Geometry: final body of the model. Coordinates: model frame, mm. A direction names the side the tool comes from. Give positions to 0.01 mm unless a question says otherwise; leave off trailing zeros. Write each loop counter-clockwise with the first axis right and the second up, starting at its lowest first coordinate (ties: lowest second). Pieces come first, ordered by that corner, then holes. Notation, with made-up numbers: (68, 47) -> (102, 47) arc R33 cw to (102, 83) -> close; hole circle Ø8 at (34.5, 2). An arc over 180 degrees is marked (long way). Use CSV: the item, a comma, the result in double quotes. Start each with the question number.
1) Set-up query: faces 1 (the face through (14, 5, 2)), 2 (the face through (2, 27.42, 2)), 3 (the face through (26, 19.42, 2)), 4 (the face through (19.5, 35, 2)), 5 (the face through (8, 35, 2)). Return all of +Z, -Z, +X, -X, +Y, -Y with unobstructed straight access to the full face (end or side cutting, diameter ignored); none if empty.
2) Section C-C (z = 3). Output: boundary loops of the cut face in (x, y), plus the area to 3 significant figures.
3) Section A-A (y = 19). Output: boundary loops of the cut face in (x, z).
4) Material intervals for line 1 (Y direction, x = 13.75, z = 2.6); line 2 (Y direction, x = 24.49, z = 1.7); line 3 (X direction, y = 14.5, z = 3.65), sorted ascending. Write a range as [from, to].
5) Section D-D (x = 4.5). Output: boundary loops of the cut face in (y, z), plus the area to 3 significant figures.
6) Contact query for flat-ended pins moving along their axis: P1, Ø2, axis at x = 2.5, z = 2.5, coming from the -Y side; P2, Ø1, axis at x = 24.5, z = 1, coming from the +Y side; P3, Ø2, axis at y = 35, z = 1.5, coming from the -X side. Output: stop coordinate, or through.
7) Section B-B (x = 24). Output: boundary loops of the cut face in (y, z), plus the area to 3 significant figures.
8) Draft query along Y for faces 6 (the face through (4, 32.42, 2)), 7 (the face through (2, 2.1, 2)), 8 (the face through (2, 19.42, 2)), 9 (the face through (25, 27.42, 2)). Return one class per face: pulls with the +Y half, pulls with the -Y half, needs draft (parallel to the pull), parting line crosses it, or undercut.
```python
from build123d import *

# Parameters (mm, degrees)
SKETCH1_R           = 1.2
SKETCH1_W           = 12.42
SKETCH1_H           = 22.42
BOSS_EXTRUDE1_DEPTH = 4
FILLET1_R           = 7


with BuildPart() as part:
    # Sketch1 → Boss-Extrude1 (new body)
    with BuildSketch(Plane.XY):
        Polygon((8, 37.42), (8, 32.42), (0, 32.42), (0, 27.42), (4, 27.42), (4, 19.42), (0, 19.42), (0, 0), (27.5, 0), (27.5, 19.42), (23.5, 19.42), (23.5, 27.42), (27.5, 27.42), (27.5, 32.42), (19.5, 32.42), (19.5, 37.42), align=None)
        with Locations((4, 13)):
            Circle(SKETCH1_R, mode=Mode.SUBTRACT)
        with Locations((13.75, 16.21)):
            Rectangle(SKETCH1_W, SKETCH1_H, mode=Mode.SUBTRACT)
        with Locations((24.49, 13.01)):
            Circle(SKETCH1_R, mode=Mode.SUBTRACT)
        with Locations((13.75, 34.42)):
            Circle(SKETCH1_R, mode=Mode.SUBTRACT)
    extrude(amount=BOSS_EXTRUDE1_DEPTH)

    # Fillet1
    fillet1_edges = [part.edges().sort_by_distance(p)[0] for p in [
        (27.5, 0, 2),
        (0, 0, 2),
    ]]
    fillet(fillet1_edges, radius=FILLET1_R)


solid = part.part
```
Answers follow:
1,face 1,"+Z, -Z"
1,face 2,"+Z, -Z, -X"
1,face 3,"+Z, -Z, +X"
1,face 4,"+Z, -Z, +X, +Y"
1,face 5,"+Z, -Z, -X, +Y"
2,outline,"(0, 7) arc R7 ccw to (7, 0) -> (20.5, 0) arc R7 ccw to (27.5, 7) -> (27.5, 19.42) -> (23.5, 19.42) -> (23.5, 27.42) -> (27.5, 27.42) -> (27.5, 32.42) -> (19.5, 32.42) -> (19.5, 37.42) -> (8, 37.42) -> (8, 32.42) -> (0, 32.42) -> (0, 27.42) -> (4, 27.42) -> (4, 19.42) -> (0, 19.42) -> close; hole circle Ø2.4 at (4, 13); hole (7.54, 5) -> (19.96, 5) -> (19.96, 27.42) -> (7.54, 27.42) -> close; hole circle Ø2.4 at (13.75, 34.42); hole circle Ø2.4 at (24.49, 13.01)"
2,area,"572 mm^2"
3,outline,"(0, 0) -> (7.54, 0) -> (7.54, 4) -> (0, 4) -> close; (19.96, 0) -> (27.5, 0) -> (27.5, 4) -> (19.96, 4) -> close"
4,line 1,"y = [0, 5], [27.42, 33.22], [35.62, 37.42]"
4,line 2,"y = [1.25, 11.81], [14.21, 19.42], [27.42, 32.42]"
4,line 3,"x = [0, 7.54], [19.96, 27.5]"
5,outline,"(0.46, 0) -> (11.91, 0) -> (11.91, 4) -> (0.46, 4) -> close; (14.09, 0) -> (32.42, 0) -> (32.42, 4) -> (14.09, 4) -> close"
5,area,"119 mm^2"
6,P1,"stops at y = 0.94"
6,P2,"stops at y = 32.42"
6,P3,"stops at x = 8"
7,outline,"(0.94, 0) -> (11.91, 0) -> (11.91, 4) -> (0.94, 4) -> close; (14.11, 0) -> (19.42, 0) -> (19.42, 4) -> (14.11, 4) -> close; (27.42, 0) -> (32.42, 0) -> (32.42, 4) -> (27.42, 4) -> close"
7,area,"85.2 mm^2"
8,face 6,"pulls with the +Y half"
8,face 7,"pulls with the -Y half"
8,face 8,"undercut"
8,face 9,"undercut"
